from build123d import *

# Parameters (mm, degrees)
SKETCH005_R       = 41.5
SKETCH005_R_2     = 12.75
PAD001_DEPTH      = 16.5
CYLINDER003_R     = 16
CYLINDER003_DEPTH = 25.2
CYLINDER008_R     = 4
CYLINDER008_DEPTH = 25
CYLINDER009_R     = 4
CYLINDER009_DEPTH = 25
POCKET_START      = -1.25
SKETCH084_R       = 48
SKETCH084_R_2     = 40
POCKET_DEPTH      = 14


with BuildPart() as part:
    # Sketch005 → Pad001 (new body)
    with BuildSketch(Plane.XY):
        with Locations((0, -21.25)):
            Circle(SKETCH005_R)
        Circle(SKETCH005_R_2, mode=Mode.SUBTRACT)
        with BuildLine():
            ThreePointArc((-31.480397, -26.993223), (-24.225688, -42.15732), (-10.285714, -51.551882))
            ThreePointArc((-10.285714, -51.551882), (-6.670071, -51.015521), (-5, -47.764147))
            Line((-5, -27.568098), (-5, -47.764147))
            ThreePointArc((-5, -27.568098), (-5.762291, -25.219217), (-7.758621, -23.765601))
            ThreePointArc((-16.637158, -18.660251), (-12.462129, -21.672456), (-7.758621, -23.765601))
            ThreePointArc((-16.637158, -18.660251), (-27.032318, -17.53007), (-31.480397, -26.993223))
        make_face(mode=Mode.SUBTRACT)
        with BuildLine():
            ThreePointArc((10.285714, -51.551882), (24.225688, -42.15732), (31.480397, -26.993223))
            ThreePointArc((31.480397, -26.993223), (27.032318, -17.53007), (16.637158, -18.660251))
            ThreePointArc((7.758621, -23.765601), (12.462129, -21.672456), (16.637158, -18.660251))
            ThreePointArc((7.758621, -23.765601), (5.762291, -25.219217), (5, -27.568098))
            Line((5, -27.568098), (5, -47.764147))
            ThreePointArc((5, -47.764147), (6.670071, -51.015521), (10.285714, -51.551882))
        make_face(mode=Mode.SUBTRACT)
    extrude(amount=-PAD001_DEPTH)

    # Cylinder003 → Cylinder003 (cut)
    with BuildSketch(Plane.XY.offset(-14)):
        Circle(CYLINDER003_R)
    extrude(amount=CYLINDER003_DEPTH, mode=Mode.SUBTRACT)

    # Cylinder008 → Cylinder008 (cut)
    with BuildSketch(Plane(origin=(23, 0, -13), x_dir=(1, 0, 0), z_dir=(0, 0, 1))):
        Circle(CYLINDER008_R)
    extrude(amount=CYLINDER008_DEPTH, mode=Mode.SUBTRACT)

    # Cylinder009 → Cylinder009 (cut)
    with BuildSketch(Plane(origin=(-23, 0, -13), x_dir=(1, 0, 0), z_dir=(0, 0, 1))):
        Circle(CYLINDER009_R)
    extrude(amount=CYLINDER009_DEPTH, mode=Mode.SUBTRACT)

    # Sketch084 → Pocket (cut)
    with BuildSketch(Plane.XY.offset(POCKET_START)):
        with Locations((0, -21.25)):
            Circle(SKETCH084_R)
        with Locations((0, -21.25)):
            Circle(SKETCH084_R_2, mode=Mode.SUBTRACT)
    extrude(amount=-POCKET_DEPTH, mode=Mode.SUBTRACT)


solid = part.part
Build history of the part. All positions in model axes, mm. A direction names the side the tool comes from. Round coordinates to 2 decimals unless told otherwise and drop trailing zeros. Loops run counter-clockwise (first coordinate to the right, second up) from the corner with the lowest first, then second, coordinate; pieces in that order, holes last. Notation, with made-up numbers: (69.5, -3) -> (120.5, -3) arc R19 ccw to (120.5, 14) -> close; hole circle Ø1 at (42.25, 65.25). An arc over 180 degrees is marked (long way). Use CSV: the item, a comma, the result in double quotes. Start each with the question number.
Q1. Which spindle directions (+Z, -Z, +X, -X, +Y, -Y) get a long thin tool onto all of the face, cutting with end or side? Do faces 4 (the face through (-1, -21, -16.5)), 5 (the face through (6.627, -50.984, -8.134)), 6 (the face through (19, 0, -7)). Say none if no direction does.
Q2. Drill centre lines: L1, parallel to Y at x = 0, z = -6.75; L2, parallel to X at y = 0, z = -5; L3, parallel to Y at x = -8, z = -4.75. Where is each one in solid material? Low to high.
Q3. Saw through at D-D on y = -6.5. Give the cut face in (x, z).
Q4. Flat gauge pins, fed straight in: pin 1 Ø6 at (y, z) = (-9.5, -9) entering from +X; pin 2 Ø8 at (y, z) = (9.5, -3) entering from +X; pin 3 Ø1.5 at (y, z) = (-42, -2.5) entering from -X. Where does each tip first touch, or does it go through?
Q5. Saw through at A-A on z = -5.5. Give the cut face in (x, y), and give its area (3 significant figures).
Q6. Mould opens along X. For faces 1 (the face through (-22, 13, -15.25)), 2 (the face through (5, -38, -8)), 3 (the face through (-8.67, -60.3, -8.15)) say: +X half, -X half, draft (parallel to the pull), parting line (faces both ways), or undercut.
Q7. Saw through at C-C on y = -26. Give the cut face in (x, z).
Q8. Saw through at B-B on x = 0. Give the cut face in (y, z).
Solutions:
1,face 4,"-Z, +X, -X, +Y, -Y"
1,face 5,"+Z, -Z"
1,face 6,"+Z"
2,L1,"y = -61.25 to -16, 16 to 18.75"
2,L2,"x = -33.89 to -27, -19 to -16, 16 to 19, 27 to 33.89"
2,L3,"y = -60.44 to -51.64, -23.69 to -13.86, 13.86 to 17.94"
3,outline,"(-38.79, -16.5) -> (-10.97, -16.5) -> (-10.97, -14) -> (-14.62, -14) -> (-14.62, 0) -> (-38.79, 0) -> (-38.79, -1.25) -> (-37.18, -1.25) -> (-37.18, -15.25) -> (-38.79, -15.25) -> close; (10.97, -16.5) -> (38.79, -16.5) -> (38.79, -15.25) -> (37.18, -15.25) -> (37.18, -1.25) -> (38.79, -1.25) -> (38.79, 0) -> (14.62, 0) -> (14.62, -14) -> (10.97, -14) -> close"
4,pin 1,"stops at x = 39.03"
4,pin 2,"stops at x = 31.38"
4,pin 3,"stops at x = -34.64"
5,outline,"circle Ø80 at (0, -21.25); hole (-31.48, -26.99) arc R32 ccw to (-10.29, -51.55) arc R4 ccw to (-5, -47.76) -> (-5, -27.57) arc R4 ccw to (-7.76, -23.77) arc R25 cw to (-16.64, -18.66) arc R9 ccw to start; hole circle Ø8 at (-23, 0); hole circle Ø32 at (0, 0); hole (5, -47.76) arc R4 ccw to (10.29, -51.55) arc R32 ccw to (31.48, -26.99) arc R9 ccw to (16.64, -18.66) arc R25 cw to (7.76, -23.77) arc R4 ccw to (5, -27.57) -> close; hole circle Ø8 at (23, 0)"
5,area,"2,770 mm^2"
6,face 1,"draft"
6,face 2,"undercut"
6,face 3,"parting line"
7,outline,"(-41.23, -16.5) -> (-31.61, -16.5) -> (-31.61, 0) -> (-41.23, 0) -> (-41.23, -1.25) -> (-39.72, -1.25) -> (-39.72, -15.25) -> (-41.23, -15.25) -> close; (-5.32, -16.5) -> (5.32, -16.5) -> (5.32, 0) -> (-5.32, 0) -> close; (31.61, -16.5) -> (41.23, -16.5) -> (41.23, -15.25) -> (39.72, -15.25) -> (39.72, -1.25) -> (41.23, -1.25) -> (41.23, 0) -> (31.61, 0) -> close"
8,outline,"(-62.75, -16.5) -> (-12.75, -16.5) -> (-12.75, -14) -> (-16, -14) -> (-16, 0) -> (-62.75, 0) -> (-62.75, -1.25) -> (-61.25, -1.25) -> (-61.25, -15.25) -> (-62.75, -15.25) -> close; (12.75, -16.5) -> (20.25, -16.5) -> (20.25, -15.25) -> (18.75, -15.25) -> (18.75, -1.25) -> (20.25, -1.25) -> (20.25, 0) -> (16, 0) -> (16, -14) -> (12.75, -14) -> close"
